Geometry: final body of the model. Coordinates: model frame, mm. Round coordinates to 2 decimals unless told otherwise and drop trailing zeros. Write each loop counter-clockwise with the first axis right and the second up, starting at its lowest first coordinate (ties: lowest second). Pieces come first, ordered by that corner, then holes. Notation, with made-up numbers: M 0,10 L 17,10 A28 ccw 17,34 Z; hole C -22,15 d2. An arc over 180 degrees is marked long. Answer as CSV lines item,"result". Start each with the question number.
Q1. Section query C-C on x = -109.5. Output: boundary loops of the cut face in (y, z), and give its area (3 significant figures).
Q2. First-contact query: pin 1 (1.5 mm diameter, centred on y = -364.5, z = 3.5, fed in from -X); pin 2 (1 mm diameter, centred on x = 124.5, z = 4.5, fed in from -Y); pin 3 (7.5 mm diameter, centred on x = 196.88, y = -341, fed in from -Z); pin 4 (1 mm diameter, centred on x = 12.5, z = 3, fed in from +Y). Flat tips, straight axial feed; report the tip coordinate or a pass-through.
Q3. Section query B-B on x = 85. Output: boundary loops of the cut face in (y, z), and give its area (3 significant figures).
Q4. Mould query, pull axis X, two halves, no side actions, for faces 1 (the cylindrical face through (-186.53, -317.945, 2.88)), 2 (the flat face through (3, -352, 0)), 3 (the flat face through (-214.402, -345.955, 2.88)). Classes: pulls with the +X half, pulls with the -X half, needs draft (parallel to the pull), parting line crosses it, or undercut.
Q5. Section query A-A on z = 4.5. Give the number of separate pieces and of enclosed holes in the cut face, and give its area (3 significant figures).
Q6. Ray query, probe 1 along X at (y, z) = (-353.5, 5.45); probe 2 along X at (y, z) = (-350, 2.95); probe 3 along Y at (x, z) = (1, 2.85). Return the intervals inside material, ascending.
```python
from build123d import *

# Parameters (mm, degrees)
SKETCH1_R           = 3.175
BOSS_EXTRUDE1_DEPTH = 5.842
FILLET1_R           = 6.35


with BuildPart() as part:
    # Sketch1 → Boss-Extrude1 (new body)
    with BuildSketch(Plane.XY):
        with BuildLine():
            Line((-226.924230888, -367.644297366), (-214.224230888, -345.64725211))
            Line((-214.224230888, -345.64725211), (-201.524230888, -323.650206854))
            ThreePointArc((-201.524230888, -323.650206854), (-182.614690973, -320.065127313), (-181.873832769, -339.29725211))
            Line((-181.873832769, -339.29725211), (181.873832769, -339.29725211))
            ThreePointArc((181.873832769, -339.29725211), (182.614690973, -320.065127313), (201.524230888, -323.650206854))
            Line((201.524230888, -323.650206854), (214.224230888, -345.64725211))
            Line((214.224230888, -345.64725211), (226.924230888, -367.644297366))
            ThreePointArc((226.924230888, -367.644297366), (226.046266682, -381.666604531), (212.782184711, -386.299103732))
            ThreePointArc((212.782184711, -386.299103732), (0, -359.548814266), (-212.782184711, -386.299103732))
            ThreePointArc((-212.782184711, -386.299103732), (-226.046266682, -381.666604531), (-226.924230888, -367.644297366))
        make_face()
        with Locations((-203.22570826, -351.99725211)):
            Circle(SKETCH1_R, mode=Mode.SUBTRACT)
        with Locations((-209.57570826, -362.995774738)):
            Circle(SKETCH1_R, mode=Mode.SUBTRACT)
        with Locations((-215.92570826, -373.994297366)):
            Circle(SKETCH1_R, mode=Mode.SUBTRACT)
        with Locations(Location((196.87570826, -340.998729482, 0), (0, 0, 180))):
            Circle(SKETCH1_R, mode=Mode.SUBTRACT)
        with Locations(Location((203.22570826, -351.99725211, 0), (0, 0, 180))):
            Circle(SKETCH1_R, mode=Mode.SUBTRACT)
        with Locations(Location((209.57570826, -362.995774738, 0), (0, 0, 180))):
            Circle(SKETCH1_R, mode=Mode.SUBTRACT)
        with Locations(Location((215.92570826, -373.994297366, 0), (0, 0, 180))):
            Circle(SKETCH1_R, mode=Mode.SUBTRACT)
        with Locations((-196.87570826, -340.998729482)):
            Circle(SKETCH1_R, mode=Mode.SUBTRACT)
        with Locations((-190.52570826, -330.000206854)):
            Circle(SKETCH1_R, mode=Mode.SUBTRACT)
        with Locations(Location((190.52570826, -330.000206854, 0), (0, 0, 180))):
            Circle(SKETCH1_R, mode=Mode.SUBTRACT)
    extrude(amount=BOSS_EXTRUDE1_DEPTH)

    # Fillet1
    fillet1_edges = [part.edges().sort_by_distance(p)[0] for p in [
        (-181.873832769, -339.29725211, 2.921),
        (181.873832769, -339.29725211, 2.921),
    ]]
    fillet(fillet1_edges, radius=FILLET1_R)


solid = part.part
```
Entries:
1,outline,"M -366.55,0 L -339.3,0 L -339.3,5.84 L -366.55,5.84 Z"
1,area,"159 mm^2"
2,pin 1,"stops at x = -225.54"
2,pin 2,"stops at y = -368.69"
2,pin 3,"stops at z = 0"
2,pin 4,"stops at y = -339.3"
3,outline,"M -363.76,0 L -339.3,0 L -339.3,5.84 L -363.76,5.84 Z"
3,area,"143 mm^2"
4,face 1,"undercut"
4,face 2,"needs draft"
4,face 3,"pulls with the -X half"
5,separate pieces,"1"
5,enclosed holes,"10"
5,area,"14,000 mm^2"
6,probe 1,"x = -218.76 to -206.02, -200.43 to 200.43, 206.02 to 218.76"
6,probe 2,"x = -216.74 to -205.69, -200.76 to 200.76, 205.69 to 216.74"
6,probe 3,"y = -359.55 to -339.3"
